Model file for the job. Use its own axes, mm. Face numbers are marked on the shaded views. Round coordinates to 2 decimals unless told otherwise and drop trailing zeros. Order: outer loops, then holes, each group sorted by start corner. A loop starts at its lowest first (then second) coordinate and runs counter-clockwise, first axis right, second up. Notation, with made-up numbers: M -31.5,79.5 L -23.5,79.5 A23 ccw -23.5,109.5 Z; hole C 23,39 d4. An arc over 180 degrees is marked long. Return JSON: item names as keys, results as strings. Group by question number.
Item 1: Slice it at B-B on y = 23.5. Write the cut outline in (x, z), then the cut area to 3 significant figures.
Item 2: Pin check, flat tips, straight feed: pin 1 Ø0.8 at (y, z) = (22, 7) entering from +X; pin 2 Ø3 at (y, z) = (41.5, 8) entering from -X; pin 3 Ø3 at (x, y) = (-7.5, 11.5) entering from -Z. Stop position of each tip, or through.
Item 3: Pull direction X, two halves, no side cores. Call the marked faces 1, 2 and 3: pulls with the +X half, pulls with the -X half, needs draft (parallel to the pull), parting line crosses it, or undercut.
Item 4: Slice it at C-C on z = 10.5. Write the cut outline in (x, y), then the cut area to 3 significant figures.
Item 5: Slice it at D-D on x = 0.5. Write the cut outline in (y, z), then the cut area to 3 significant figures.
Item 6: Slice it at A-A on z = 8.5. Write the cut outline in (x, y).
Item 7: Probe line 1 along X through (y, z) = (29.5, 8.5); line 2 along X through (y, z) = (32.5, 11.5); line 3 along X through (y, z) = (47, 10.25). List the from-to ranges inside material, lowest first.
Autodesk Fusion 360 part; units mm, degrees
sketch "Sketch1" plane through (0, 0, 0) normal (0, 1, 0) x (1, 0, 0)
  line L0 (10, -10) -> (-10, -10)
  line L1 (-10, -10) -> (-10, 10)
  line L2 (-10, 10) -> (10, 10)
  line L3 (10, 10) -> (10, -10)
  line L4 (10, -10) -> (-10, 10) construction
  line L5 (-10, -10) -> (10, 10) construction
  line L6 (-10, -10) -> (10, -10)
  line L7 (10, -10) -> (10, -13)
  line L8 (10, -13) -> (-10, -13)
  line L9 (-10, -13) -> (-10, -10)
  line L10 (-3.75, -13) -> (-3.75, 10)
  line L11 (3.75, -13) -> (3.75, 10)
  line L12 (-2.95, -13) -> (-2.95, 10)
  line L13 (2.95, -13) -> (2.95, 10)
  line L14 (6, -13) -> (6, 10)
  line L15 (-6, 10) -> (-6, -13)
  line L16 (-10, -8) -> (10, -8)
  line L17 (-2.25, -13) -> (-2.25, 10)
  line L18 (2.25, -13) -> (2.25, 10)
  line L19 (10, -6.5) -> (-10, -6.5)
  line L20 (10, -12.2) -> (-10, -12.2)
  line L21 (6, -12.2) -> (9.182, -12.2) construction
  line L22 (6.3314, -13) -> (10.913, -13) construction
  line L23 (-6, -12.2) -> (-9.182, -12.2) construction
  line L24 (-6.3314, -13) -> (-10.9441, -13) construction
  line L25 (2.95, -8) -> (3.75, -7.2)
  line L26 (2.95, -8) -> (4.0607, -8) construction
  line L27 (2.95, -6.5) -> (3.75, -7.2)
  line L28 (-2.95, -8) -> (-3.75, -7.2)
  line L29 (-2.95, -8) -> (-4.0607, -8) construction
  line L30 (-2.95, -6.5) -> (-3.75, -7.2)
  line L31 (-10, -10) -> (-7, -13)
  line L32 (-10, -10) -> (-5.7574, -10) construction
  line L33 (-8.8686, -10) -> (-6.6686, -12.2)
  line L34 (10, -10) -> (7, -13)
  line L35 (10, -10) -> (5.7574, -10) construction
  line L36 (8.8686, -10) -> (6.6686, -12.2)
  line L37 (3.35, -8) -> (3.35, -6.5)
  line L38 (-3.35, -8) -> (-3.35, -6.5)
  dimension "d1" = 20
  dimension "d2" = 20
  dimension "d3" = 20
  dimension "d4" = 3
  dimension "d5" = 7.5
  dimension "d6" = 3.75
  dimension "d7" = 5.9
  dimension "d8" = 2.95
  dimension "d9" = 12
  dimension "d10" = 6
  dimension "d11" = 2
  dimension "d12" = 4.5
  dimension "d13" = 2.25
  dimension "d14" = 1.5
  dimension "d15" = 0.8
  dimension "d29" = 45
  dimension "d30" = 45
  dimension "d31" = 45
  dimension "d32" = 45
  dimension "d33" = 0.8
  dimension "d34" = 0.8
  dimension "d35" = 0.4
  dimension "d36" = 0.4
extrude "Extrude1" add sketch "Sketch1" along normal blind 50 contours L0 L6 L20 L34 L36 | L8 L14 L20 L34 | L8 L11 L14 L20 | L0 L6 L13 L18 L20 | L0 L6 L13 L16 L18 | L8 L11 L13 L20 | L8 L13 L18 L20 | L13 L16 L18 L19 | L13 L25 L27 L37 | L0 L6 L12 L17 L20 | L0 L6 L12 L16 L17 | L8 L17 L18 L20 | L8 L12 L17 L20 | L12 L16 L17 L19 | L8 L10 L12 L20 | L12 L28 L30 L38 | L8 L10 L15 L20 | L0 L6 L20 L31 L33 | L8 L15 L20 L31
chamfer "Chamfer5" distance 0.5 angle 45 4 edges at (-2.25, 25, 12.2) (-2.95, 25, 12.2) (2.25, 25, 12.2) (2.95, 25, 12.2)
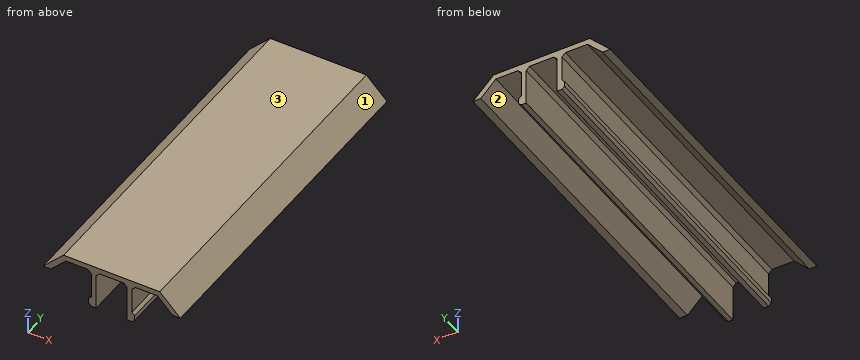
Output values:
{
 "1": {"outline": "M -10,10 L -8.87,10 L -6.67,12.2 L -3.45,12.2 L -2.95,11.7 L -2.95,8 L -3.35,7.6 L -3.35,6.85 L -2.95,6.5 L -2.25,6.5 L -2.25,11.7 L -1.75,12.2 L 1.75,12.2 L 2.25,11.7 L 2.25,6.5 L 2.95,6.5 L 3.35,6.85 L 3.35,7.6 L 2.95,8 L 2.95,11.7 L 3.45,12.2 L 6.67,12.2 L 8.87,10 L 10,10 L 7,13 L -7,13 Z", "area": "26.2 mm²"},
 "2": {"pin 1": "x = 3.35", "pin 2": "x = -3.35", "pin 3": "z = 10"},
 "3": {"face 1": "pulls with the +X half", "face 2": "undercut", "face 3": "needs draft"},
 "4": {"outline": "M -9.5,0 L -8.37,0 L -8.37,50 L -9.5,50 Z; M -2.95,0 L -2.25,0 L -2.25,50 L -2.95,50 Z; M 2.25,0 L 2.95,0 L 2.95,50 L 2.25,50 Z; M 8.37,0 L 9.5,0 L 9.5,50 L 8.37,50 Z", "area": "183 mm²"},
 "5": {"outline": "M 0,12.2 L 50,12.2 L 50,13 L 0,13 Z", "area": "40.0 mm²"},
 "6": {"outline": "M -2.95,0 L -2.25,0 L -2.25,50 L -2.95,50 Z; M 2.25,0 L 2.95,0 L 2.95,50 L 2.25,50 Z"},
 "7": {"line 1": "-2.95 to -2.25, 2.25 to 2.95", "line 2": "-8.5 to -7.37, -2.95 to -2.25, 2.25 to 2.95, 7.37 to 8.5", "line 3": "-9.75 to -8.62, -2.95 to -2.25, 2.25 to 2.95, 8.62 to 9.75"}
}
